The listing builds one solid part. Answer for the finished solid, in the listing's coordinates (mm). A direction names the side the tool comes from. Give positions to 0.01 mm unless a question says otherwise; leave off trailing zeros. Write each loop counter-clockwise with the first axis right and the second up, starting at its lowest first coordinate (ties: lowest second). Pieces come first, ordered by that corner, then holes. Notation, with made-up numbers: (68, 48) -> (105, 48) arc R26 ccw to (105, 67) -> close; hole circle Ø5 at (69, -2). An arc over 180 degrees is marked (long way). Write each question's results on one line, items separated by ' | '. Start each with the question number.
Autodesk Inventor part; units mm, degrees
ref_plane "YZ Plane" through (0, 0, 0) normal (1, 0, 0) x (0, 1, 0)
ref_plane "XZ Plane" through (0, 0, 0) normal (0, 1, 0) x (-1, 0, 0)
ref_plane "XY Plane" through (0, 0, 0) normal (0, 0, 1) x (1, 0, 0)
sketch "Sketch1" plane through (0, 0, 0) normal (0, 1, 0) x (-1, 0, 0)
  line L0 (0, 0) -> (199.9996, 0)
  line L1 (199.9996, 0) -> (199.9996, -310.5912)
  line L2 (199.9996, -310.5912) -> (0, -310.5912)
  line L3 (0, -310.5912) -> (0, 0)
  dimension "d0" = 199.9996
  dimension "d1" = 310.5912
extrude "Extrusion1" add sketch "Sketch1" along normal blind 24.9936
sketch "Sketch2" plane through (0, 24.9936, 0) normal (0, 1, 0) x (1, 0, 0)
  circle A0 centre (-174.5996, 25.4) radius 6.35
  circle A1 centre (-174.5996, 285.1912) radius 6.35
  circle A2 centre (-25.4, 25.4) radius 6.35
  circle A3 centre (-25.4, 285.1912) radius 6.35
  line L0 (-199.9996, 310.5912) -> (-199.9996, 0)
  line L1 (-199.9996, 0) -> (0, 0)
  line L2 (0, 310.5912) -> (-199.9996, 310.5912)
  line L3 (0, 0) -> (0, 310.5912)
  dimension "d4" = 12.7
  dimension "d5" = 25.4
  dimension "d6" = 25.4
  dimension "d7" = 12.7
  dimension "d8" = 25.4
  dimension "d9" = 25.4
  dimension "d10" = 25.4
  dimension "d11" = 25.4
  dimension "d12" = 12.7
  dimension "d13" = 12.7
  dimension "d14" = 25.4
  dimension "d15" = 25.4
extrude "Extrusion2" cut sketch "Sketch2" against normal blind 24.9936 contours A0 | A1 | A2 | A3
sketch "Sketch3" plane through (-199.9996, 0, 0) normal (0, 0, 1) x (1, 0, 0)
  circle A0 centre (50, 12.4968) radius 6.35
  circle A1 centre (149.9996, 12.4968) radius 6.35
  line L0 (0, 0) -> (0, 24.9936)
  line L1 (0, 24.9936) -> (199.9996, 24.9936)
  line L2 (199.9996, 0) -> (199.9996, 24.9936)
  point P0 (199.9996, 12.4968)
  dimension "d18" = 12.7
  dimension "d19" = 50
  dimension "d20" = 12.4968
  dimension "d21" = 12.4968
  dimension "d22" = 50
  dimension "d23" = 12.7
sketch "Sketch4" plane through (0, 0, -310.5912) normal (0, 0, -1) x (-1, 0, 0)
  circle A0 centre (50, 12.4968) radius 6.35
  circle A1 centre (149.9996, 12.4968) radius 6.35
  line L0 (0, 0) -> (0, 24.9936)
  line L1 (0, 0) -> (199.9996, 0)
  line L2 (199.9996, 0) -> (199.9996, 24.9936)
  dimension "d24" = 12.7
  dimension "d25" = 12.7
  dimension "d26" = 50
  dimension "d27" = 12.4968
  dimension "d28" = 12.4968
  dimension "d29" = 50
extrude "Extrusion3" cut sketch "Sketch3" against normal blind 20
extrude "Extrusion4" cut sketch "Sketch4" against normal blind 20
equation "\"d7\" = d4"
equation "\"d8\" = d5"
equation "\"d9\" = d5"
equation "\"d10\" = d5"
equation "\"d11\" = d5"
equation "\"d12\" = d4"
equation "\"d13\" = d4"
equation "\"d14\" = d5"
equation "\"d15\" = d5"
equation "\"d21\" = d20"
equation "\"d23\" = d18"
equation "\"d24\" = d18"
equation "\"d25\" = d18"
equation "\"d26\" = d22"
equation "\"d27\" = d21"
equation "\"d28\" = d21"
equation "\"d29\" = d26"
properties part number "FloorMountV2"
1. A tool of negligible diameter and unlimited length cuts with its end or side. For faces 1 (the cylindrical face through (-56.344, 12.776, -9.86)), 2 (the flat face through (-50, 13, -290.591)), 3 (the flat face through (-99, 12, 0)), from which of +Z, -Z, +X, -X, +Y, -Y can it reach the whole face along a straight path? Write none if from no direction.
2. Section B-B (z = -25.4) is taken. Write down the section's boundary in (x, y).
3. Section D-D (x = -149) is taken. Write down the section's boundary in (y, z).
4. Consider probe 1 along Z at (x, y) = (-26.5, 13.25); probe 2 along X at (y, z) = (4.5, -27.5); probe 3 along Z at (x, y) = (-171, 1.75). Determine where each line is inside the solid, lowest interval first. Write a range as [from, to].
5. Each of these flat-tipped pins is pushed along its axis until it touches: pin 1 Ø10 at (x, z) = (-25.4, -25.4) entering from -Y; pin 2 Ø8 at (x, z) = (-148, -90) entering from -Y; pin 3 Ø10 at (x, y) = (-50, 12.5) entering from +Z; pin 4 Ø4 at (x, y) = (-49.5, 10.5) entering from -Z. Where does it stop, or does it pass through?
6. The mould has two halves that part along Y. Classify faces 4 (the cylindrical face through (-156.343, 12.776, -9.86)), 5 (the flat face through (-99, 0, -153)), 6 (the flat face through (0, 12, -157)): pulls with the +Y half, pulls with the -Y half, needs draft (parallel to the pull), parting line crosses it, or undercut.
7. Section A-A (x = -25.4) is taken. Write down the section's boundary in (y, z).
8. Section C-C (x = -50) is taken. Write down the section's boundary in (y, z), then the cut area to 3 significant figures.
Results:
1) face 1: +Z | face 2: -Z | face 3: +Z, +X, -X, +Y, -Y
2) outline: (-200, 0) -> (-180.95, 0) -> (-180.95, 24.99) -> (-200, 24.99) -> close; (-168.25, 0) -> (-31.75, 0) -> (-31.75, 24.99) -> (-168.25, 24.99) -> close; (-19.05, 0) -> (0, 0) -> (0, 24.99) -> (-19.05, 24.99) -> close
3) outline: (0, -310.59) -> (6.23, -310.59) -> (6.23, -290.59) -> (18.77, -290.59) -> (18.77, -310.59) -> (24.99, -310.59) -> (24.99, 0) -> (18.77, 0) -> (18.77, -20) -> (6.23, -20) -> (6.23, 0) -> (0, 0) -> close
4) probe 1: z = [-310.59, -291.45], [-278.94, -31.65], [-19.15, 0] | probe 2: x = [-200, -180.59], [-168.61, -31.39], [-19.41, 0] | probe 3: z = [-310.59, -290.42], [-279.96, -30.63], [-20.17, 0]
5) pin 1: passes through | pin 2: stops at y = 0 | pin 3: stops at z = -20 | pin 4: stops at z = -290.59
6) face 4: undercut | face 5: pulls with the -Y half | face 6: needs draft
7) outline: (0, -310.59) -> (24.99, -310.59) -> (24.99, -291.54) -> (0, -291.54) -> close; (0, -278.84) -> (24.99, -278.84) -> (24.99, -31.75) -> (0, -31.75) -> close; (0, -19.05) -> (24.99, -19.05) -> (24.99, 0) -> (0, 0) -> close
8) outline: (0, -310.59) -> (6.15, -310.59) -> (6.15, -290.59) -> (18.85, -290.59) -> (18.85, -310.59) -> (24.99, -310.59) -> (24.99, 0) -> (18.85, 0) -> (18.85, -20) -> (6.15, -20) -> (6.15, 0) -> (0, 0) -> close | area: 7,250 mm²
